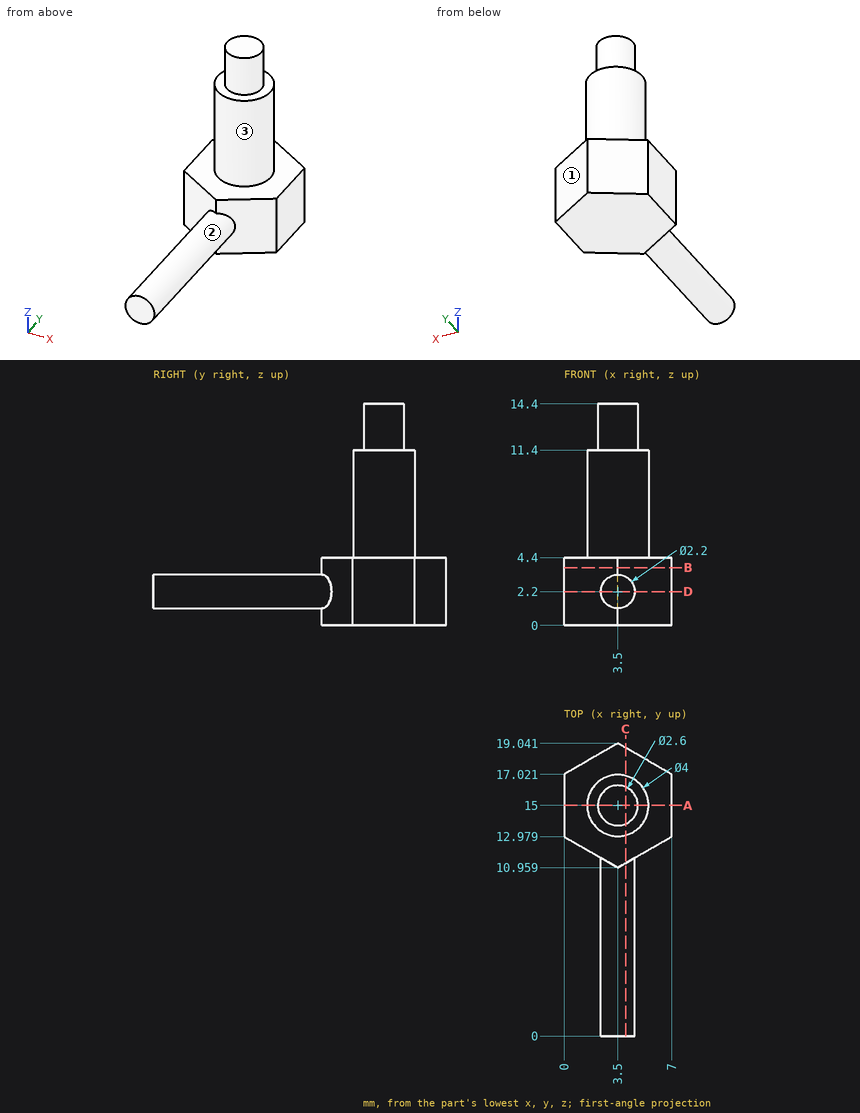
Verification items for this drawing (mm, ordinates from the low corner). A direction names the side the tool comes from. Coordinates: 2 decimals unless noted, no trailing zeros. Loops run counter-clockwise (first coordinate to the right, second up) from the corner with the lowest first, then second, coordinate; pieces in that order, holes last. Notation, with made-up numbers: (23.25, 85.25) -> (66.25, 85.25) arc R22 cw to (66.25, 106.25) -> close; hole circle Ø2 at (8.5, 51.5). An arc over 180 degrees is marked (long way). Answer in a Markdown table with one row per item. Add a question column.
1. Access from +Z, -Z, +X, -X, +Y, -Y to the whole of each face (thin tool, end or side, straight path). Record for the marked faces 1, 2 and 3.
2. Section check C-C, the plane x = 4. Enter the section's corners in (y, z).
3. Section check A-A, the plane y = 15. Enter the section's corners in (x, z).
4. Material ranges on probe 1 along Z at (x, y) = (0.5, 14.25); probe 2 along Z at (x, y) = (3.5, 7.75); probe 3 along Y at (x, z) = (2.5, 7.25), recorded low to high. Write a range as [from, to].
5. Section check D-D, the plane z = 2.2. Enter the section's corners in (x, y).
6. Depth check by flat-ended pin: P1, Ø3, axis at y = 6, z = 4.5, coming from the -X side (1 decimal); P2, Ø1.5, axis at x = 1, z = 11, coming from the +Y side. Enter the tip coordinate at first touch or a pass-through.
7. Section check B-B, the plane z = 3.75. Enter the section's corners in (x, y).
Derived:
| question | item | result |
|---|---|---|
| 1 | face 1 | +Z, -Z, +X, +Y |
| 1 | face 2 | -Y |
| 1 | face 3 | +Z |
| 2 | outline | (0, 1.22) -> (11.25, 1.22) -> (11.25, 0) -> (18.75, 0) -> (18.75, 4.4) -> (16.94, 4.4) -> (16.94, 11.4) -> (16.2, 11.4) -> (16.2, 14.4) -> (13.8, 14.4) -> (13.8, 11.4) -> (13.06, 11.4) -> (13.06, 4.4) -> (11.25, 4.4) -> (11.25, 3.18) -> (0, 3.18) -> close |
| 3 | outline | (0, 0) -> (7, 0) -> (7, 4.4) -> (5.5, 4.4) -> (5.5, 11.4) -> (4.8, 11.4) -> (4.8, 14.4) -> (2.2, 14.4) -> (2.2, 11.4) -> (1.5, 11.4) -> (1.5, 4.4) -> (0, 4.4) -> close |
| 4 | probe 1 | z = [0, 4.4] |
| 4 | probe 2 | z = [1.1, 3.3] |
| 4 | probe 3 | y = [13.27, 16.73] |
| 5 | outline | (0, 12.98) -> (2.4, 11.59) -> (2.4, 0) -> (4.6, 0) -> (4.6, 11.59) -> (7, 12.98) -> (7, 17.02) -> (3.5, 19.04) -> (0, 17.02) -> close |
| 6 | P1 | stops at x = 2.7 |
| 6 | P2 | stops at y = 15.97 |
| 7 | outline | (0, 12.98) -> (3.5, 10.96) -> (7, 12.98) -> (7, 17.02) -> (3.5, 19.04) -> (0, 17.02) -> close |
